Verification items for this drawing (mm, ordinates from the low corner). A direction names the side the tool comes from. Round coordinates to 2 decimals unless told otherwise and drop trailing zeros. Loops run counter-clockwise (first coordinate to the right, second up) from the corner with the lowest first, then second, coordinate; pieces in that order, holes last. Notation, with made-up numbers: (36, -11.5) -> (57, -11.5) arc R9 ccw to (57, -5.5) -> close; hole circle Ø8 at (14.5, 27). An arc over 180 degrees is marked (long way). Use a Markdown table: item, result. Add a question column.
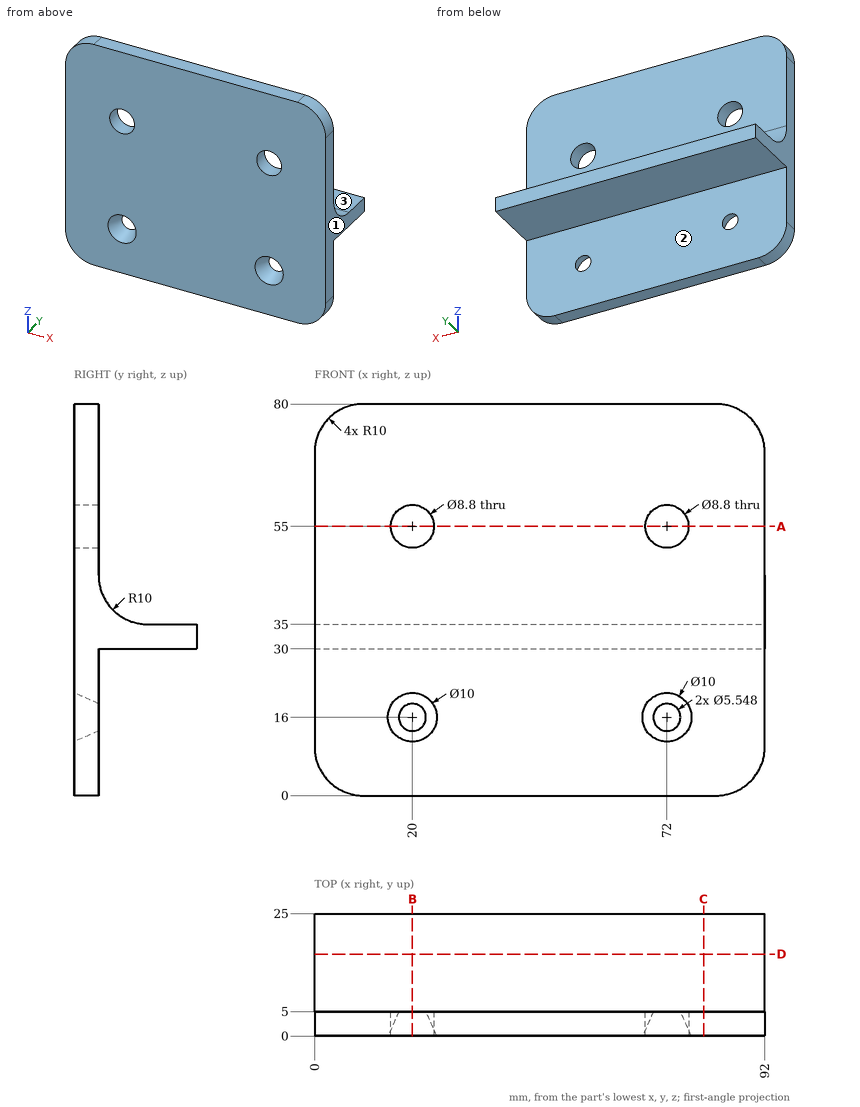
1) Go/stop test with flat-tipped pins: pin 1 (12 mm diameter, centred on x = 49, y = 21.5, fed in from +Z); pin 2 (10.5 mm diameter, centred on x = 49, z = 60, fed in from +Y); pin 3 (11 mm diameter, centred on x = 64.5, y = 19.5, fed in from +Z). Record where each tip stops, or that it passes through.
2) Sectioned sample at D-D on y = 16.75. Enter the section's corners in (x, z).
3) Sectioned sample at A-A on z = 55. Enter the section's corners in (x, y), then the cut area to 3 significant figures.
4) Sectioned sample at C-C on x = 79.5. Enter the section's corners in (y, z).
5) Thickness scan on line 1 (X direction, y = 2.3, z = 55); line 2 (Z direction, x = 72, y = 3.55); line 3 (Z direction, x = 20, y = 2.7). Record the ranges inside material, lowest first.
6) Sectioned sample at B-B on x = 20. Enter the section's corners in (y, z).
7) Access from +Z, -Z, +X, -X, +Y, -Y to the whole of each face (thin tool, end or side, straight path). Record for the marked faces 1, 2 and 3.
Geometry results:
| question | item | result |
|---|---|---|
| 1 | pin 1 | z = 35 |
| 1 | pin 2 | y = 5 |
| 1 | pin 3 | z = 35.05 |
| 2 | outline | (0, 30) -> (92, 30) -> (92, 35) -> (0, 35) -> close |
| 3 | outline | (0, 0) -> (15.6, 0) -> (15.6, 5) -> (0, 5) -> close; (24.4, 0) -> (67.6, 0) -> (67.6, 5) -> (24.4, 5) -> close; (76.4, 0) -> (92, 0) -> (92, 5) -> (76.4, 5) -> close |
| 3 | area | 372 mm^2 |
| 4 | outline | (0, 0) -> (5, 0) -> (5, 30) -> (25, 30) -> (25, 35) -> (15, 35) arc R10 cw to (5, 45) -> (5, 80) -> (0, 80) -> close |
| 5 | line 1 | 0 to 15.6, 24.4 to 67.6, 76.4 to 92 |
| 5 | line 2 | 0 to 12.58, 19.42 to 50.6, 59.4 to 80 |
| 5 | line 3 | 0 to 12.2, 19.8 to 50.6, 59.4 to 80 |
| 6 | outline | (0, 0) -> (5, 0) -> (5, 13.23) -> (0, 11) -> close; (0, 21) -> (5, 18.77) -> (5, 30) -> (25, 30) -> (25, 35) -> (15, 35) arc R10 cw to (5, 45) -> (5, 50.6) -> (0, 50.6) -> close; (0, 59.4) -> (5, 59.4) -> (5, 80) -> (0, 80) -> close |
| 7 | face 1 | +Z, -Z, +X, +Y, -Y |
| 7 | face 2 | -Z, +X, -X, +Y |
| 7 | face 3 | +Z, +X, -X, +Y |
